Part model, mm, in its own coordinate system. Face numbers are marked on the shaded views. A direction names the side the tool comes from. Give positions to 0.01 mm unless a question says otherwise; leave off trailing zeros. Loops run counter-clockwise (first coordinate to the right, second up) from the corner with the lowest first, then second, coordinate; pieces in that order, holes last. Notation, with made-up numbers: M -5.75,86.25 L 8.25,86.25 A24 ccw 8.25,106.25 Z; hole C 85,61 d7. An arc over 180 degrees is marked long. Put each result on its own line as item: value. Start each with the question number.
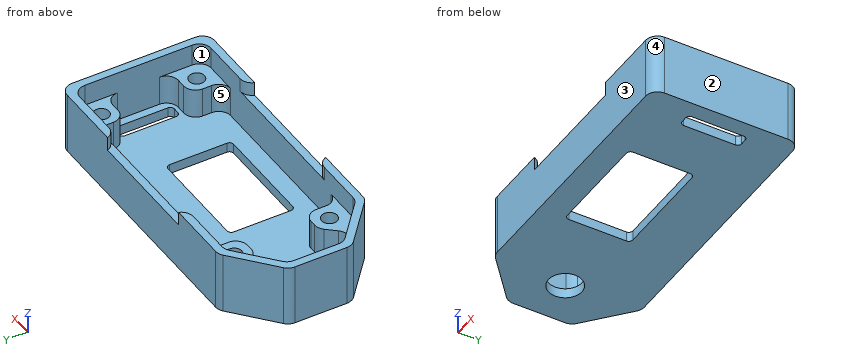
```python
from build123d import *

# Parameters (mm, degrees)
BOSS_EXTRUDE1_DEPTH = 19.999999999999996
CUT_EXTRUDE1_DEPTH  = 17.5
CUT_EXTRUDE2_DEPTH  = 20
BOSS_EXTRUDE2_DEPTH = 7.5
SKETCH5_R           = 1.949999999999999
SKETCH5_R_2         = 1.949999999999998
SKETCH5_R_3         = 1.9499999999999986
CUT_EXTRUDE3_DEPTH  = 5.5
SKETCH6_R           = 4.199999999999999
CUT_EXTRUDE4_DEPTH  = 10
CUT_EXTRUDE5_DEPTH  = 2.5
CUT_EXTRUDE10_DEPTH = 7.5
SKETCH13_W          = 78.99999999999999
SKETCH13_H          = 37
CUT_EXTRUDE11_DEPTH = 4.5
CUT_EXTRUDE12_DEPTH = 3.5
SKETCH9_W           = 3.5
SKETCH9_H           = 15.000000000000004
CUT_EXTRUDE7_DEPTH  = 2.5
FILLET2_R           = 3
FILLET18_R          = 3
FILLET19_R          = 3
FILLET11_R          = 3
FILLET12_R          = 1
FILLET14_R          = 3
FILLET15_R          = 3
FILLET13_R          = 1
FILLET20_R          = 3


with BuildPart() as part:
    # Sketch1 → Boss-Extrude1 (new body)
    with BuildSketch(Plane.XY):
        Polygon((0, 0), (78.99999999999999, 0), (78.99999999999999, 37), (-6.72e-15, 37), align=None)
    extrude(amount=-BOSS_EXTRUDE1_DEPTH)

    # Sketch2 → Cut-Extrude1 (cut)
    with BuildSketch(Plane.XY):
        Polygon((76.99999999999999, 34.99999999999999), (12.999999999999984, 34.99999999999999), (1.9999999999999831, 25.499999999999996), (1.9999999999999718, 11.5), (13.000000000000004, 1.9999999999999922), (76.99999999999999, 2.0000000000000004), align=None)
    extrude(amount=-CUT_EXTRUDE1_DEPTH, mode=Mode.SUBTRACT)

    # Sketch3 → Cut-Extrude2 (cut)
    with BuildSketch(Plane.XY):
        Polygon((12.255906978158162, 37), (-6.72e-15, 26.41535306431793), (0, 37), align=None)
        Polygon((12.255906978158176, 1e-17), (1.389e-14, 10.584646935682041), (0, 0), align=None)
    extrude(amount=-CUT_EXTRUDE2_DEPTH, mode=Mode.SUBTRACT)

    # Sketch4 → Boss-Extrude2 (add)
    with BuildSketch(Plane.XY.offset(-17.5)):
        Polygon((76.99999999999999, 34.99999999999999), (68.74999999999999, 34.99999999999999), (68.74999999999999, 26.75), (76.99999999999997, 26.75), align=None)
        Polygon((12.999999999999984, 34.99999999999999), (20.49999999999999, 34.99999999999999), (20.49999999999999, 1.9999999999999922), (13.000000000000004, 1.9999999999999922), (1.9999999999999896, 11.49999999999998), (1.9999999999999882, 25.49999999999998), align=None)
        Polygon((76.99999999999999, 2), (68.74999999999999, 2.000000000000003), (68.74999999999999, 10.249999999999996), (76.99999999999999, 10.249999999999998), align=None)
    extrude(amount=BOSS_EXTRUDE2_DEPTH)

    # Sketch5 → Cut-Extrude3 (cut)
    with BuildSketch(Plane.XY.offset(-10.000000000000002)):
        with Locations((16.499999999999986, 30.5)):
            Circle(SKETCH5_R)
        with Locations((72.49999999999999, 30.5)):
            Circle(SKETCH5_R_2)
        with Locations((72.49999999999999, 6.499999999999999)):
            Circle(SKETCH5_R_3)
        with Locations((16.499999999999986, 6.499999999999985)):
            Circle(SKETCH5_R)
    extrude(amount=-CUT_EXTRUDE3_DEPTH, mode=Mode.SUBTRACT)

    # Sketch6 → Cut-Extrude4 (cut)
    with BuildSketch(Plane.XY.offset(-10.000000000000002)):
        with Locations((10.999999999999988, 18.5)):
            Circle(SKETCH6_R)
    extrude(amount=-CUT_EXTRUDE4_DEPTH, mode=Mode.SUBTRACT)

    # Sketch7 → Cut-Extrude5 (cut)
    with BuildSketch(Plane.XY.offset(-17.5)):
        Polygon((30.999999999999986, 23), (57.99999999999998, 23.000000000000004), (57.99999999999998, 6.500000000000003), (30.99999999999999, 6.499999999999999), align=None)
    extrude(amount=-CUT_EXTRUDE5_DEPTH, mode=Mode.SUBTRACT)

    # Sketch12 → Cut-Extrude10 (cut)
    with BuildSketch(Plane.XY.offset(-10.000000000000002)):
        Polygon((9.751406193775388, 32.19439625826063), (14.669293871364125, 26.5), (20.49999999999999, 26.5), (20.499999999999993, 10.499999999999986), (14.669293871364117, 10.499999999999986), (9.751406193775411, 4.805603741739363), (2.000000000000001, 11.499999999999991), (1.9999999999999862, 25.499999999999975), align=None)
    extrude(amount=-CUT_EXTRUDE10_DEPTH, mode=Mode.SUBTRACT)

    # Sketch13 → Cut-Extrude11 (cut)
    with BuildSketch(Plane.XY):
        with Locations((39.49999999999999, 18.5)):
            Rectangle(SKETCH13_W, SKETCH13_H)
    extrude(amount=-CUT_EXTRUDE11_DEPTH, mode=Mode.SUBTRACT)

    # Sketch14 → Cut-Extrude12 (cut)
    with BuildSketch(Plane.XY.offset(-4.5)):
        Polygon((28.999999999999986, 37), (58.999999999999986, 37.00000000000001), (58.999999999999986, 35), (28.999999999999986, 34.99999999999999), align=None)
        Polygon((28.999999999999986, 1.9999999999999931), (58.999999999999986, 1.9999999999999987), (58.999999999999986, 0), (28.999999999999986, -5.51e-15), align=None)
    extrude(amount=-CUT_EXTRUDE12_DEPTH, mode=Mode.SUBTRACT)

    # Sketch9 → Cut-Extrude7 (cut)
    with BuildSketch(Plane.XY.offset(-17.5)):
        with Locations((73.24999999999999, 18.75)):
            Rectangle(SKETCH9_W, SKETCH9_H)
    extrude(amount=-CUT_EXTRUDE7_DEPTH, mode=Mode.SUBTRACT)

    # Fillet2
    fillet2_edges = [part.edges().sort_by_distance(p)[0] for p in [
        (76.99999999999997, 26.75, -13.75),
        (68.74999999999999, 34.99999999999999, -13.75),
        (20.49999999999999, 1.9999999999999922, -13.75),
        (20.49999999999999, 34.99999999999999, -13.75),
        (76.99999999999999, 10.249999999999998, -13.75),
        (68.74999999999999, 2.000000000000003, -13.75),
    ]]
    fillet(fillet2_edges, radius=FILLET2_R)

    # Fillet18
    fillet18_edges = [part.edges().sort_by_distance(p)[0] for p in [
        (20.499999999999993, 10.499999999999986, -13.750000000000002),
        (20.49999999999999, 26.5, -13.750000000000002),
        (68.74999999999999, 26.75, -13.75),
        (68.74999999999999, 10.249999999999996, -13.75),
    ]]
    fillet(fillet18_edges, radius=FILLET18_R)

    # Fillet19
    fillet19_edges = [part.edges().sort_by_distance(p)[0] for p in [
        (9.751406193775411, 4.805603741739363, -13.750000000000002),
        (14.669293871364117, 10.499999999999986, -13.750000000000002),
        (14.669293871364125, 26.5, -13.750000000000002),
        (9.751406193775388, 32.19439625826063, -13.750000000000002),
    ]]
    fillet(fillet19_edges, radius=FILLET19_R)

    # Fillet11
    fillet11_edges = [part.edges().sort_by_distance(p)[0] for p in [
        (-6.72e-15, 26.41535306431793, -12.25),
        (12.255906978158162, 37, -12.25),
        (1.389e-14, 10.584646935682041, -12.25),
        (12.255906978158176, 1e-17, -12.25),
        (78.99999999999999, 37, -12.249999999999998),
        (78.99999999999999, 0, -12.249999999999998),
    ]]
    fillet(fillet11_edges, radius=FILLET11_R)

    # Fillet12
    fillet12_edges = [part.edges().sort_by_distance(p)[0] for p in [
        (57.99999999999998, 6.500000000000003, -18.75),
        (57.99999999999998, 23.000000000000004, -18.75),
        (30.999999999999986, 23, -18.75),
        (30.99999999999999, 6.499999999999999, -18.75),
    ]]
    fillet(fillet12_edges, radius=FILLET12_R)

    # Fillet14
    # the kernel refuses this fillet: 3 mm, written as the material it takes off along each edge
    with BuildSketch(Plane(origin=(58.999999999999986, 1.9999999999999982, 2.5710678118654613), x_dir=(-3.55e-15, -1, 0), z_dir=(0, 0, -1))) as fillet14_piece_1:
        with BuildLine():
            CenterArc((2.99999999999999, -2.828427124746195), FILLET14_R, 109.47122063449055, 70.52877936550925)
            Line((-1.027e-14, -2.8284271247461845), (-0.0600000000000101, -2.8284271247461845))
            Line((-0.0600000000000101, -2.8284271247461845), (-0.06000000000000005, 2.1e-16))
            Line((-0.06000000000000005, 2.1e-16), (2.1e-16, 0.06000000000000227))
            ThreePointArc((2.1e-16, 0.06000000000000227), (0.9999999999999986, 0.05999999999999872), (1.9799999999999969, 0.05656854249492234))
            Line((1.9799999999999969, 0.05656854249492234), (1.9999999999999967, 0))
        make_face()
    extrude(amount=10.571067811865461, mode=Mode.SUBTRACT)
    with BuildSketch(Plane(origin=(28.999999999999986, 1.9999999999999942, 2.571067811865479), x_dir=(0, -1, 0), z_dir=(0, 0, -1))) as fillet14_piece_2:
        with BuildLine():
            CenterArc((3, 2.8284271247461916), FILLET14_R, 180, 70.52877936550931)
            Line((2.2e-16, 2.8284271247461916), (-0.05999999999999961, 2.8284271247461916))
            Line((-0.05999999999999961, 2.8284271247461916), (-0.06000000000000005, 0))
            Line((-0.06000000000000005, 0), (0, -0.05999999999999872))
            ThreePointArc((0, -0.05999999999999872), (1.0000000000000002, -0.05999999999999872), (1.9800000000000004, -0.05656854249492227))
            Line((1.9800000000000004, -0.05656854249492227), (2.0000000000000004, 0))
        make_face()
    extrude(amount=10.571067811865479, mode=Mode.SUBTRACT)
    with BuildSketch(Plane(origin=(58.999999999999986, 34.99999999999999, 2.571067811865479), x_dir=(0, 1, 0), z_dir=(0, 0, -1))) as fillet14_piece_3:
        with BuildLine():
            CenterArc((3, 2.8284271247461916), FILLET14_R, 180, 70.52877936550954)
            Line((0, 2.8284271247461916), (-0.06000000000000227, 2.8284271247461916))
            Line((-0.06000000000000227, 2.8284271247461916), (-0.06000000000000227, 0))
            Line((-0.06000000000000227, 0), (0, -0.06000000000000227))
            ThreePointArc((0, -0.06000000000000227), (1.000000000000007, -0.06000000000000227), (1.980000000000011, -0.05656854249492227))
            Line((1.980000000000011, -0.05656854249492227), (2.000000000000014, 0))
        make_face()
    extrude(amount=10.571067811865479, mode=Mode.SUBTRACT)
    with BuildSketch(Plane(origin=(28.999999999999986, 34.99999999999999, 2.571067811865479), x_dir=(0, 1, 0), z_dir=(0, 0, -1))) as fillet14_piece_4:
        with BuildLine():
            CenterArc((3, -2.8284271247461916), FILLET14_R, 109.47122063449056, 70.52877936550944)
            Line((0, -2.8284271247461916), (-0.06000000000000227, -2.8284271247461916))
            Line((-0.06000000000000227, -2.8284271247461916), (-0.06000000000000227, 0))
            Line((-0.06000000000000227, 0), (0, 0.05999999999999872))
            ThreePointArc((0, 0.05999999999999872), (1.000000000000007, 0.05999999999999872), (1.980000000000004, 0.05656854249492227))
            Line((1.980000000000004, 0.05656854249492227), (2.000000000000007, 0))
        make_face()
    extrude(amount=10.571067811865479, mode=Mode.SUBTRACT)

    # Fillet15
    fillet15_edges = [part.edges().sort_by_distance(p)[0] for p in [
        (76.99999999999999, 34.99999999999999, -7.25),
        (12.999999999999984, 34.99999999999999, -7.25),
        (13.000000000000004, 1.9999999999999922, -7.25),
        (76.99999999999999, 2.0000000000000004, -7.25),
    ]]
    fillet(fillet15_edges, radius=FILLET15_R)

    # Fillet13
    fillet13_edges = [part.edges().sort_by_distance(p)[0] for p in [
        (74.99999999999999, 11.25, -18.75),
        (74.99999999999999, 26.25, -18.75),
        (71.49999999999999, 26.25, -18.75),
        (71.49999999999999, 11.25, -18.75),
    ]]
    fillet(fillet13_edges, radius=FILLET13_R)

    # Fillet20
    fillet20_edges = [part.edges().sort_by_distance(p)[0] for p in [
        (1.9999999999999851, 25.499999999999982, -11),
        (1.99999999999999, 11.499999999999995, -11),
    ]]
    fillet(fillet20_edges, radius=FILLET20_R)


solid = part.part
```
1) Mould opens along X. For the marked faces 1, 2 and 3 say: +X half, -X half, draft (parallel to the pull), parting line (faces both ways), or undercut.
2) Wall check: L1, parallel to Y at x = 72.5, z = -11.6; L2, parallel to X at y = 13.5, z = -18.25; L3, parallel to Y at x = 16.5, z = -11.4. Give the ranges that are in metal, low to high.
3) Which spindle directions (+Z, -Z, +X, -X, +Y, -Y) get a long thin tool onto all of the face, cutting with end or side? Do the marked faces 4 and 5. Say none if no direction does.
4) Pin check, flat tips, straight feed: pin 1 Ø12 at (x, y) = (70, 6) entering from +Z; pin 2 Ø1.1 at (y, z) = (30.5, -14.5) entering from -X; pin 3 Ø1.5 at (x, y) = (38, 21.5) entering from +Z; pin 4 Ø5 at (x, y) = (9, 20) entering from +Z. Stop position of each tip, or through.
5) Band-saw the part on C-C on z = -10.75. State how many separate pieces and enclosed holes the cut face has, then the cut area to 3 significant figures.
6) Band-saw the part on B-B on x = 25. Give the cut face in (y, z).
Evaluation:
1. face 1: undercut
1. face 2: +X half
1. face 3: draft
2. L1: 0 to 4.55, 8.45 to 10.25, 26.75 to 28.55, 32.45 to 37
2. L2: 0 to 31, 58 to 71.5, 75 to 79
2. L3: 0 to 4.55, 8.45 to 10.5, 26.5 to 28.55, 32.45 to 37
3. face 4: +Z, -Z, +X, -Y
3. face 5: +Z
4. pin 1: z = -4.5
4. pin 2: x = 4.09
4. pin 3: through
4. pin 4: z = -17.5
5. separate pieces: 1
5. enclosed holes: 5
5. area: 660 mm2
6. outline: M 0,-20 L 37,-20 L 37,-4.5 L 35,-4.5 L 35,-17.5 L 2,-17.5 L 2,-4.5 L 0,-4.5 Z
